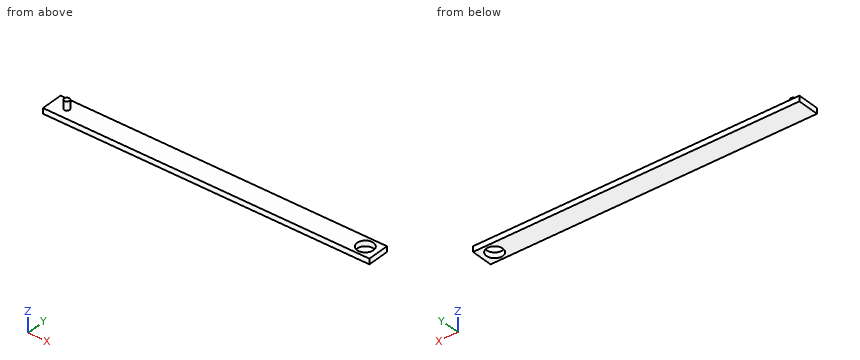
```python
from build123d import *

# Parameters (mm, degrees)
SKETCH1_W           = 300
SKETCH1_H           = 20
BOSS_EXTRUDE1_DEPTH = 5
SKETCH2_R           = 7.5
CUT_EXTRUDE1_DEPTH  = 151.416089565
SKETCH3_R           = 2.5
BOSS_EXTRUDE2_DEPTH = 8


with BuildPart() as part:
    # Sketch1 → Boss-Extrude1 (new body)
    with BuildSketch(Plane.XY):
        Rectangle(SKETCH1_W, SKETCH1_H)
    extrude(amount=BOSS_EXTRUDE1_DEPTH)

    # Sketch2 → Cut-Extrude1 (cut, through all)
    with BuildSketch(Plane.XY.offset(5)):
        with Locations((138.172978114, 0)):
            Circle(SKETCH2_R)
    extrude(amount=-CUT_EXTRUDE1_DEPTH, mode=Mode.SUBTRACT)

    # Sketch3 → Boss-Extrude2 (add)
    with BuildSketch(Plane.XY.offset(5)):
        with Locations((-136.185092233, 0)):
            Circle(SKETCH3_R)
    extrude(amount=BOSS_EXTRUDE2_DEPTH)


solid = part.part
```
Work out the finished part from the listing and answer in its coordinate system (mm). Give positions to 0.01 mm unless a question says otherwise; leave off trailing zeros. Write each loop counter-clockwise with the first axis right and the second up, starting at its lowest first coordinate (ties: lowest second). Pieces come first, ordered by that corner, then holes. Notation, with made-up numbers: (57, -18.5) -> (73, -18.5) arc R23 cw to (73, -1.5) -> close; hole circle Ø6 at (19.5, 51). An arc over 180 degrees is marked (long way). Write item = value, one per line.
Q1. Flat-ended cylindrical pins translate along their axes: pin 1 Ø12 at (x, y) = (138.17, 0) entering from -Z; pin 2 Ø10 at (x, y) = (32.5, 3.5) entering from +Z; pin 3 Ø2 at (y, z) = (0.5, 8.5) entering from -X. Find the tip coordinate at first contact, or state that the pin passes through.
Computed values:
pin_1 = through
pin_2 = 5
pin_3 = -138.69
Q2. Section B-B on z = 2.75 is taken. Determine the outline of the cut face in (x, y), and give its area (3 significant figures).
Computed values:
outline = (-150, -10) -> (150, -10) -> (150, 10) -> (-150, 10) -> close; hole circle Ø15 at (138.17, 0)
area = 5,820 mm^2
Q3. Section C-C on x = -78 is taken. Determine the outline of the cut face in (y, z).
Computed values:
outline = (-10, 0) -> (10, 0) -> (10, 5) -> (-10, 5) -> close
Q4. Section A-A on y = 0 is taken. Determine the outline of the cut face in (x, z), and give its area (4 significant figures).
Computed values:
outline = (-150, 0) -> (130.67, 0) -> (130.67, 5) -> (-133.69, 5) -> (-133.69, 13) -> (-138.69, 13) -> (-138.69, 5) -> (-150, 5) -> close; (145.67, 0) -> (150, 0) -> (150, 5) -> (145.67, 5) -> close
area = 1,465 mm^2
Q5. Consider line 1 along X through (y, z) = (0.75, 1.5); line 2 along Z through (x, y) = (-21.5, -8.5); line 3 along X through (y, z) = (-4.75, 3.5). Determine where each line is inside the solid, lowest interval first.
Computed values:
line_1 = -150 to 130.71, 145.64 to 150
line_2 = 0 to 5
line_3 = -150 to 132.37, 143.98 to 150
